Study the drawing (mm; zero at the part's minimum x, y, z) and answer. A direction names the side the tool comes from. Give positions to 0.01 mm unless a question says otherwise; leave off trailing zeros. Order: outer loops, then holes, each group sorted by start corner. A loop starts at its lowest first (then second) coordinate and runs counter-clockwise, first axis right, second up. Notation, with made-up numbers: (1.25, 67) - (42.25, 67) arc R29 cw to (42.25, 101) - close; hole circle Ø5 at (17.5, -17.75). An arc over 180 degrees is marked (long way). Use CSV: the item, a comma, the result in double quotes.
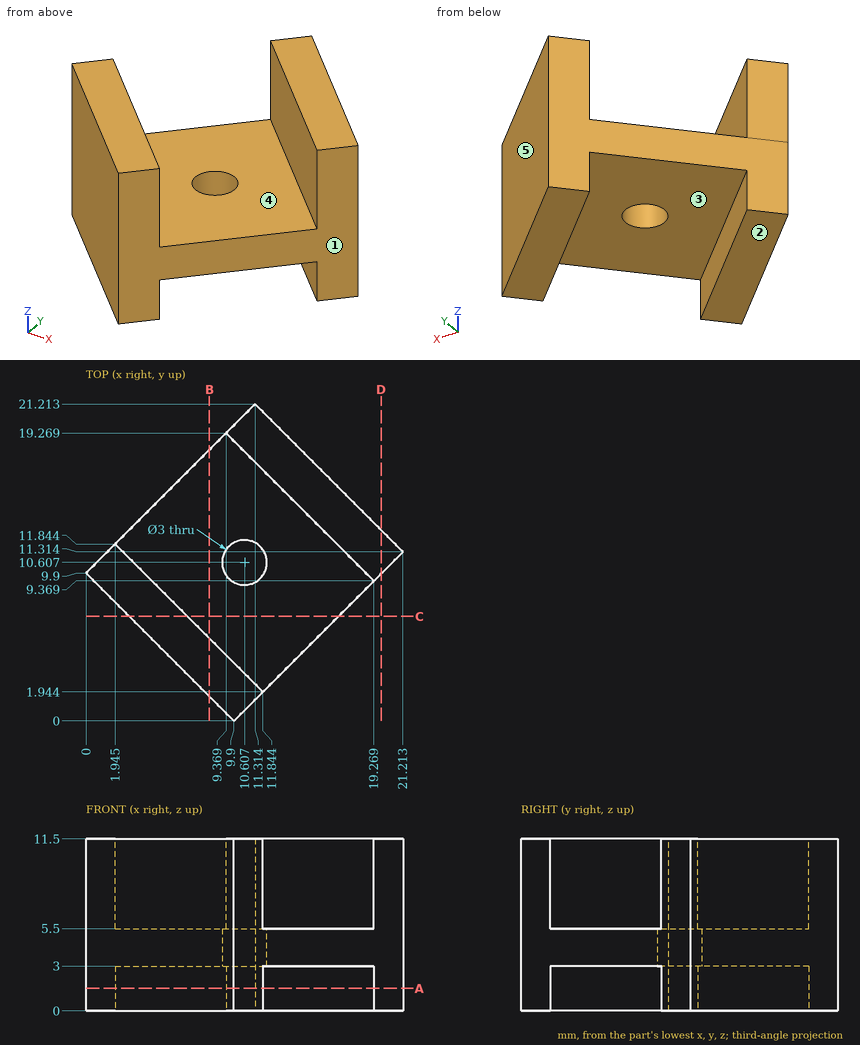
Item 1: The part is cut by section D-D (x = 19.75). Give the vertices of the cut face in (y, z).
Taken from the geometry:
outline,"(9.85, 0) - (12.78, 0) - (12.78, 11.5) - (9.85, 11.5) - close"
Item 2: Each of these flat-tipped pins is pushed along its axis until it touches: pin 1 (2 mm diameter, centred on x = 14.5, y = 13.5, fed in from -Z); pin 2 (3 mm diameter, centred on x = 4, z = 4.5, fed in from +Y); pin 3 (5 mm diameter, centred on y = 5, z = 4, fed in from +X); pin 4 (5 mm diameter, centred on x = 15, y = 7, fed in from +Z). Where does it stop, or does it pass through?
Taken from the geometry:
pin 1,"z = 0"
pin 2,"y = 15.4"
pin 3,"x = 17.4"
pin 4,"z = 5.5"
Item 3: The mould has two halves that part along Y. Classify the marked faces 1, 2 and 3: +Y half, -Y half, draft (parallel to the pull), parting line (faces both ways), or undercut.
Taken from the geometry:
face 1,"-Y half"
face 2,"draft"
face 3,"undercut"
Item 4: The part is cut by section A-A (z = 1.5). Give the vertices of the cut face in (x, y) (1 decimal).
Taken from the geometry:
outline,"(0, 9.9) - (9.9, 0) - (11.8, 1.9) - (1.9, 11.8) - close; (9.4, 19.3) - (19.3, 9.4) - (21.2, 11.3) - (11.3, 21.2) - close"
Item 5: Find the intervals of material crossed by line 1 along Z through (x, y) = (4, 10.5); line 2 along X through (y, z) = (10, 6) (1 decimal); line 3 along Y through (x, z) = (16.25, 5.75) (1 decimal), in increasing order.
Taken from the geometry:
line 1,"3 to 5.5"
line 2,"0.1 to 3.8, 18.6 to 19.9"
line 3,"12.4 to 16.3"
Item 6: The part is cut by section B-B (x = 8.25). Give the vertices of the cut face in (y, z).
Taken from the geometry:
outline,"(1.65, 0) - (5.54, 0) - (5.54, 3) - (18.15, 3) - (18.15, 5.5) - (5.54, 5.5) - (5.54, 11.5) - (1.65, 11.5) - close"
Item 7: The part is cut by section C-C (y = 7). Give the vertices of the cut face in (x, z).
Taken from the geometry:
outline,"(2.9, 0) - (6.79, 0) - (6.79, 3) - (16.9, 3) - (16.9, 5.5) - (6.79, 5.5) - (6.79, 11.5) - (2.9, 11.5) - close"
Item 8: Which of the six approach directions +Z, -Z, +X, -X, +Y, -Y give full straight-line access (tool end or side, diameter ignored) to the marked faces 4 and 5?
Taken from the geometry:
face 4,"+Z"
face 5,"+Z, -Z, +X, +Y"
